Autodesk Inventor part; units mm, degrees
ref_plane "YZ Plane" through (0, 0, 0) normal (1, 0, 0) x (0, 1, 0)
ref_plane "XZ Plane" through (0, 0, 0) normal (0, 1, 0) x (-1, 0, 0)
ref_plane "XY Plane" through (0, 0, 0) normal (0, 0, 1) x (1, 0, 0)
sketch "Sketch1" plane through (0, 0, 0) normal (0, 0, 1) x (1, 0, 0)
  circle A0 centre (0, 0) radius 2.25
  circle A1 centre (31, 0) radius 2.25
  circle A2 centre (0, 31) radius 2.25
  circle A3 centre (31, 31) radius 2.25
  circle A4 centre (15.5, 15.5) radius 12.5
  line L0 (-6, 37) -> (37, 37)
  line L1 (37, 37) -> (37, -6)
  line L2 (37, -6) -> (-6, -6)
  line L3 (-6, -6) -> (-6, 37)
  line L4 (-6, 37) -> (37, -6) construction
  line L5 (37, 37) -> (-6, -6) construction
  line L6 (-6, -6) -> (37, -6)
  line L7 (37, -6) -> (37, -34)
  line L8 (37, -34) -> (-6, -34)
  line L9 (-6, -34) -> (-6, -6)
  dimension "d3" = 4.5
  dimension "d5" = 31
  dimension "d6" = 25
  dimension "d7" = 43
  dimension "d8" = 43
  dimension "d9" = 49.5
  dimension "d10" = 31
extrude "Extrusion1" add sketch "Sketch1" against normal blind 5
sketch "Sketch2" plane through (0, 0, 0) normal (0, 0, 1) x (1, 0, 0)
  line L0 (37, -34) -> (-6, -34)
  line L1 (37, 37) -> (37, -34)
  line L2 (-6, -34) -> (37, -34)
  line L3 (37, -34) -> (37, -29)
  line L4 (37, -29) -> (-6, -29)
  line L5 (-6, -29) -> (-6, -34)
  point P0 (0, 0)
  dimension "d13" = 5
extrude "Extrusion2" add sketch "Sketch2" along normal blind 25
sketch "Sketch3" plane through (-6, -29, 0) normal (0, 1, 0) x (1, 0, 0)
  circle A0 centre (6, -10) radius 2.75
  circle A1 centre (37, -10) radius 2.75
  line L0 (0, 5) -> (0, -25)
  line L1 (0, 0) -> (0, -25)
  line L2 (43, 0) -> (43, -25)
  line L3 (0, 5) -> (43, 5)
  point P0 (6, 0)
  point P1 (0, -10)
  point P2 (0, -12.5)
  dimension "d16" = 5.5
  dimension "d17" = 31
  dimension "d23" = 6
  dimension "d24" = 15
extrude "Extrusion3" cut sketch "Sketch3" against normal blind 25
fillet "Fillet1" radius 5 1 edges at (15.5, -29, 0)
sketch "Sketch4" plane through (-6, -29, 25) normal (0, 1, 0) x (1, 0, 0)
  line L0 (0, 30) -> (0, 0)
  line L1 (0, 5) -> (43.1457, 5)
  circle A0 centre (6, 15) radius 2.75
  line L2 (0, 20) -> (43, 20)
  line L3 (0, 20) -> (0, 0)
  line L4 (43, 0) -> (0, 0)
  line L5 (43, 20) -> (43, 0)
  circle A1 centre (6, 15) radius 2.75
  circle A2 centre (37, 15) radius 2.75
  point P0 (6, 25)
  point P1 (43, 5)
  dimension "d25" = 10
extrude "Extrusion4" cut sketch "Sketch4" against normal through all contours L1 L5 L4 L0
properties part number "motor_holder"
Part model, mm, in its own coordinate system. A direction names the side the tool comes from. Round coordinates to 2 decimals unless told otherwise and drop trailing zeros. Loops run counter-clockwise (first coordinate to the right, second up) from the corner with the lowest first, then second, coordinate; pieces in that order, holes last. Notation, with made-up numbers: (20.5, 71) -> (60.5, 71) arc R18 cw to (60.5, 96) -> close; hole circle Ø11 at (-27.75, -6). An arc over 180 degrees is marked (long way). Use one line per item in the form item = value. Start each with the question number.
Item 1: Band-saw the part on A-A (x = 0). List the corners of the cut face in (y, z), plus the area to 3 significant figures.
Item 2: Drop flat-ended pins along their axis: pin 1 Ø7.5 at (x, z) = (13, 14.5) entering from +Y; pin 2 Ø8 at (x, y) = (23, 0.5) entering from +Z. Give the stop position or say it passes through.
Item 3: Two-plate mould, pull along Z, no slides. Class faces 3 (the cylindrical face through (-2.027, -31.465, 8.141)), 4 (the cylindrical face through (15, -27, 1)), 5 (the flat face through (37, -6, -2)), 6 (the flat face through (15, 2, -5)): released by +Z, released by -Z, zero draft, split by the parting line, or undercut.
Item 4: Drill centre lines: line 1 along Y through (x, z) = (31, -1.35); line 2 along X through (y, z) = (-31.9, 10); line 3 along Z through (x, y) = (31, -32.25). Where is each one in solid material? Low to high.
Item 5: Band-saw the part on C-C (y = 0). List the corners of the cut face in (x, z), plus the area to 3 significant figures.
Item 6: Band-saw the part on B-B (z = -2.5). List the corners of the cut face in (x, y).
Item 7: Band-saw the part on D-D (y = 8). List the corners of the cut face in (x, z).
Item 8: Tool access for faces 1 (the flat face through (15, 0, 0)), 2 (the cylindrical face through (32.21, 32.897, -2.465)): list every direction of +Z, -Z, +X, -X, +Y, -Y with a clear straight run to the whole face (end or side of a thin tool).
Data:
q1.outline = (-34, -5) -> (-2.25, -5) -> (-2.25, 0) -> (-24, 0) arc R5 cw to (-29, 5) -> (-29, 7.25) -> (-34, 7.25) -> close; (-34, 12.75) -> (-29, 12.75) -> (-29, 20) -> (-34, 20) -> close; (2.25, -5) -> (28.75, -5) -> (28.75, 0) -> (2.25, 0) -> close; (33.25, -5) -> (37, -5) -> (37, 0) -> (33.25, 0) -> close
q1.area = 388 mm^2
q2.pin_1 = -29
q2.pin_2 = 0
q3.face_3 = undercut
q3.face_4 = released by +Z
q3.face_5 = zero draft
q3.face_6 = released by -Z
q4.line_1 = -34 to -2.25, 2.25 to 28.75, 33.25 to 37
q4.line_2 = -6 to -2.75, 2.75 to 28.25, 33.75 to 37
q4.line_3 = -5 to 7.25, 12.75 to 20
q5.outline = (-6, -5) -> (-2.25, -5) -> (-2.25, 0) -> (-6, 0) -> close; (2.25, -5) -> (28.75, -5) -> (28.75, 0) -> (2.25, 0) -> close; (33.25, -5) -> (37, -5) -> (37, 0) -> (33.25, 0) -> close
q5.area = 170 mm^2
q6.outline = (-6, -34) -> (37, -34) -> (37, 37) -> (-6, 37) -> close; hole circle Ø4.5 at (0, 0); hole circle Ø4.5 at (0, 31); hole circle Ø25 at (15.5, 15.5); hole circle Ø4.5 at (31, 0); hole circle Ø4.5 at (31, 31)
q7.outline = (-6, -5) -> (5.5, -5) -> (5.5, 0) -> (-6, 0) -> close; (25.5, -5) -> (37, -5) -> (37, 0) -> (25.5, 0) -> close
q8.face_1 = +Z, +X, -X, +Y
q8.face_2 = +Z, -Z
